Work out the finished part from the listing and answer in its coordinate system (mm). Face numbers are marked on the shaded views. A direction names the side the tool comes from. Coordinates: 2 decimals unless noted, no trailing zeros. Order: outer loops, then holes, each group sorted by start corner. A loop starts at its lowest first (then second) coordinate and runs counter-clockwise, first axis right, second up. Notation, with made-up numbers: (55, -14.75) -> (59, -14.75) arc R13 cw to (59, 8.25) -> close; hole circle Ø7 at (0.5, 4.5). An arc over 180 degrees is marked (long way). Use one line per item in the form item = value.
from build123d import *

# Parameters (mm, degrees)
SKETCH1_R                    = 1.5
BASE_FLANGE1_DEPTH           = 2
EDGE_FLANGE1_STRIP_W         = 9.5
EDGE_FLANGE1_STRIP_H         = 2
EDGE_FLANGE1_STRIP_CUT_DEPTH = 20
EDGE_FLANGE1_DEPTH           = 20
SKETCH9_R                    = 0.75
CUT_EXTRUDE1_DEPTH           = 10
FILLET1_R                    = 3
L_EK1_SCALE                  = 2


# Sheet-metal steps are written as plain solids
with BuildPart() as part:
    # Sketch1 → Base-Flange1 (new body)
    with BuildSketch(Plane(origin=(0, 0, 0), x_dir=(1, 0, 0), z_dir=(0, 1, 0))):
        with BuildLine():
            Line((0, 7), (0, -7))
            ThreePointArc((0, -7), (0.878679656, -9.121320344), (3, -10))
            Line((3, -10), (12, -10))
            Line((12, -10), (12, 10))
            Line((12, 10), (3, 10))
            ThreePointArc((3, 10), (0.878679656, 9.121320344), (0, 7))
        make_face()
        with Locations(Location((2.72, 6, 0), (0, 0, 270))):
            Circle(SKETCH1_R, mode=Mode.SUBTRACT)
        with Locations(Location((2.72, -6, 0), (0, 0, 270))):
            Circle(SKETCH1_R, mode=Mode.SUBTRACT)
    extrude(amount=BASE_FLANGE1_DEPTH)

    # Edge-Flange1 strip (across the edge) → Edge-Flange1 strip cut (cut)
    with BuildSketch(Plane(origin=(12, 2, 10), x_dir=(-1, 0, 0), z_dir=(0, 0, -1))):
        with Locations((-2, -1)):
            Rectangle(EDGE_FLANGE1_STRIP_W, EDGE_FLANGE1_STRIP_H)
    extrude(amount=EDGE_FLANGE1_STRIP_CUT_DEPTH, mode=Mode.SUBTRACT)

    # Edge-Flange1 section (across the edge) → Edge-Flange1 (add)
    with BuildSketch(Plane(origin=(12, 2, 10), x_dir=(-1, 0, 0), z_dir=(0, 0, -1))):
        with BuildLine():
            Line((0, 0.75), (0, 6))
            Line((0, 6), (2, 6))
            Line((2, 6), (2, 0.75))
            ThreePointArc((2, 0.75), (2.219669914, 0.219669914), (2.75, 0))
            Line((2.75, 0), (2.75, -2))
            ThreePointArc((2.75, -2), (0.805456352, -1.194543648), (0, 0.75))
        make_face()
    extrude(amount=EDGE_FLANGE1_DEPTH)

    # Sketch9 → Cut-Extrude1 (cut)
    with BuildSketch(Plane.ZY.offset(-10)):
        with Locations(Location((0, 6, 0), (0, 0, 270))):
            Circle(SKETCH9_R)
    extrude(amount=-CUT_EXTRUDE1_DEPTH, mode=Mode.SUBTRACT)

    # Fillet1
    fillet1_edges = [part.edges().sort_by_distance(p)[0] for p in [
        (11, 8, 10),
        (11, 8, -10),
    ]]
    fillet(fillet1_edges, radius=FILLET1_R)


with BuildPart() as part_1:
    # Ölçek1: scaled about (7.730300008, 2.413989503, 0)
    add(part.part.scale(L_EK1_SCALE).moved(Location((-7.730300008, -2.413989503, 0))))


solid = part_1.part
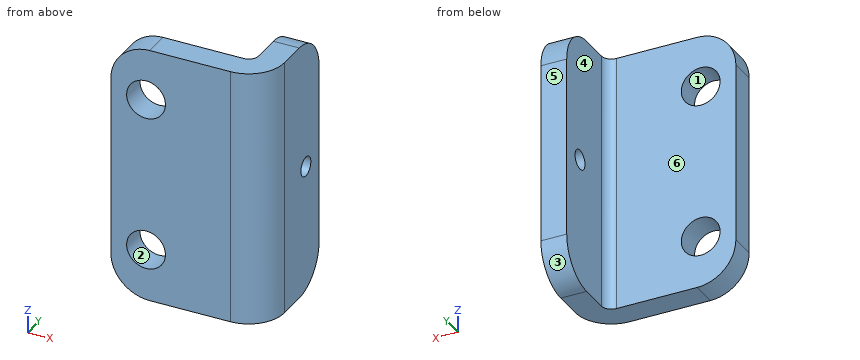
(1) Each of these flat-tipped pins is pushed along its axis until it touches: P1, Ø8, axis at x = 4, z = 15.5, coming from the +Y side; P2, Ø1, axis at y = 7, z = -1.5, coming from the -X side; P3, Ø3.5, axis at x = -2.29, z = 12, coming from the +Y side. Where does it stop, or does it pass through?
Data:
P1 = 1.59
P2 = 12.27
P3 = through
(2) Section C-C on y = 8.5 is taken. Write down the section's boundary in (x, z).
Data:
outline = (12.27, -19.93) -> (16.27, -19.93) -> (16.27, -1.03) -> (12.27, -1.03) -> close; (12.27, 1.03) -> (16.27, 1.03) -> (16.27, 19.93) -> (12.27, 19.93) -> close
(3) Straight lines are drawn through the part: line 1 along Y through (x, z) = (2, 8.5); line 2 along X through (y, z) = (-1.35, -12); line 3 along X through (y, z) = (3, 4.5). For each, find the intervals that lie inside material, in ascending order.
Data:
line_1 = -2.41 to 1.59
line_2 = -7.73 to -5.29, 0.71 to 14.02
line_3 = 12.27 to 16.27
(4) Section A-A on z = 12 is taken. Write down the section's boundary in (x, y).
Data:
outline = (-7.73, -2.41) -> (-5.29, -2.41) -> (-5.29, 1.59) -> (-7.73, 1.59) -> close; (0.71, -2.41) -> (10.77, -2.41) arc R5.5 ccw to (16.27, 3.09) -> (16.27, 13.59) -> (12.27, 13.59) -> (12.27, 3.09) arc R1.5 cw to (10.77, 1.59) -> (0.71, 1.59) -> close
(5) Section B-B on x = -3 is taken. Write down the section's boundary in (y, z).
Data:
outline = (-2.41, -19.86) -> (1.59, -19.86) -> (1.59, -14.91) -> (-2.41, -14.91) -> close; (-2.41, -9.09) -> (1.59, -9.09) -> (1.59, 9.09) -> (-2.41, 9.09) -> close; (-2.41, 14.91) -> (1.59, 14.91) -> (1.59, 19.86) -> (-2.41, 19.86) -> close
(6) Section D-D on z = 7.5 is taken. Write down the section's boundary in (x, y), plus the area to 3 significant figures.
Data:
outline = (-7.73, -2.41) -> (10.77, -2.41) arc R5.5 ccw to (16.27, 3.09) -> (16.27, 13.59) -> (12.27, 13.59) -> (12.27, 3.09) arc R1.5 cw to (10.77, 1.59) -> (-7.73, 1.59) -> close
area = 138 mm²
(7) Which of the six approach directions +Z, -Z, +X, -X, +Y, -Y give full straight-line access (tool end or side, diameter ignored) to the marked faces 5 and 6?
Data:
face_5 = +Z, -Z, +X, -X, +Y
face_6 = +Z, -Z, -X, +Y
(8) The mould has two halves that part along Z. Classify the marked faces 1, 2, 3 and 4: released by +Z, released by -Z, zero draft, split by the parting line, or undercut.
Data:
face_1 = undercut
face_2 = undercut
face_3 = released by -Z
face_4 = zero draft
